```python
from build123d import *

# Parameters (mm, degrees)
F1_DEPTH = 2.54
F2_R     = 3.175
F3_DEPTH = 2.541


with BuildPart() as f1:
    # F0 (on Front) → F1 (new body)
    with BuildSketch(Plane.XZ):
        with BuildLine():
            ThreePointArc((-101.485908, 1.260738), (-99.626036, -3.22939), (-95.135908, -5.089262))
            Line((-95.135908, -5.089262), (57.264092, -5.089262))
            ThreePointArc((57.264092, -5.089262), (61.75422, -3.22939), (63.614092, 1.260738))
            ThreePointArc((63.614092, 1.260738), (61.75422, 5.750866), (57.264092, 7.610738))
            Line((57.264092, 7.610738), (-95.135908, 7.610738))
            ThreePointArc((-95.135908, 7.610738), (-99.626036, 5.750866), (-101.485908, 1.260738))
        make_face()
    extrude(amount=F1_DEPTH)

    # F2 (on face) → F3 (cut, through all)
    with BuildSketch(Plane.XZ.offset(2.54)):
        with Locations((-95.135908, 1.260738)):
            Circle(F2_R)
        with Locations((57.264092, 1.260738)):
            Circle(F2_R)
    extrude(amount=-F3_DEPTH, mode=Mode.SUBTRACT)


solid = f1.part
```
Geometry: final body of the model. Coordinates: model frame, mm. Coordinates: 2 decimals unless noted, no trailing zeros. Write each loop counter-clockwise with the first axis right and the second up, starting at its lowest first coordinate (ties: lowest second). Pieces come first, ordered by that corner, then holes. Notation, with made-up numbers: M 80.25,87.5 L 113.25,87.5 A28 ccw 113.25,116.5 Z; hole C 34,24.5 d1. An arc over 180 degrees is marked long. Use CSV: the item, a comma, the result in double quotes. Start each with the question number.
1. First-contact query: P1, Ø1, axis at y = -1, z = 0, coming from the -X side; P2, Ø1, axis at y = -1.5, z = 5, coming from the +X side. Flat tips, straight axial feed; report the tip coordinate or a pass-through.
2. Cut plane A-A on y = -1.45. Return the cut outline in (x, z) (3 decimals).
3. Mould query, pull axis Z, two halves, no side actions, for faces 1 (the face through (-20, -1, -5.089)), 2 (the face through (54.924, -1.288, 3.407)), 3 (the face through (-20, -2.54, 1)), 4 (the face through (-98.308, -1.288, 1.4)). Classes: pulls with the +Z half, pulls with the -Z half, needs draft (parallel to the pull), parting line crosses it, or undercut.
4. Cut plane B-B on z = -0.25. Return the cut outline in (x, y).
5. Cut plane C-C on z = 6. Return the cut outline in (x, y), plus the area to 3 significant figures.
6. Ray query, probe 1 along X at (y, z) = (-0.7, 3.5); probe 2 along X at (y, z) = (-1.45, 1.75); probe 3 along X at (y, z) = (-0.65, 6.75). Return the intervals inside material, ascending.
Entries:
1,P1,"x = -101.44"
1,P2,"x = 62.73"
2,outline,"M -95.136,-5.089 L 57.264,-5.089 A6.35 ccw 57.264,7.611 L -95.136,7.611 A6.35 ccw Z; hole C -95.136,1.261 d6.35; hole C 57.264,1.261 d6.35"
3,face 1,"pulls with the -Z half"
3,face 2,"undercut"
3,face 3,"needs draft"
3,face 4,"undercut"
4,outline,"M -101.3,-2.54 L -97.93,-2.54 L -97.93,0 L -101.3,0 Z; M -92.34,-2.54 L 54.47,-2.54 L 54.47,0 L -92.34,0 Z; M 60.06,-2.54 L 63.43,-2.54 L 63.43,0 L 60.06,0 Z"
5,outline,"M -99.36,-2.54 L 61.49,-2.54 L 61.49,0 L -99.36,0 Z"
5,area,"409 mm²"
6,probe 1,"-101.08 to -97.39, -92.89 to 55.01, 59.51 to 63.21"
6,probe 2,"-101.47 to -98.27, -92 to 54.13, 60.4 to 63.6"
6,probe 3,"-98.33 to 60.46"
